Check sheet for the modelled part. Datum: model origin and axes. Units: mm. Face numbers are marked on the shaded views. A direction names the side the tool comes from. Round coordinates to 2 decimals unless told otherwise and drop trailing zeros. Order: outer loops, then holes, each group sorted by start corner. A loop starts at its lowest first (then second) coordinate and runs counter-clockwise, first axis right, second up.
(1) Tool access check on the marked faces 5, 6 and 7. Record the directions out of +Z, -Z, +X, -X, +Y, -Y that give a thin tool (end or side, any length) a straight path to the whole face; none if there is none.
(2) Depth check by flat-ended pin: pin 1 (1.6 mm diameter, centred on y = 25.5, z = 2, fed in from +X); pin 2 (10 mm diameter, centred on x = 16, y = 19.5, fed in from -Z); pin 3 (3 mm diameter, centred on x = 19, y = 28, fed in from +Z); pin 4 (1.6 mm diameter, centred on x = 7, y = -6, fed in from -Z). Enter the tip coordinate at first touch or a pass-through.
(3) Mould release check, pull along Y, two halves, no side actions. Record for the marked faces 1, 2, 3 and 4: released by +Y, released by -Y, zero draft, split by the parting line, or undercut.
(4) Sectioned sample at D-D, the plane z = 7.25. Enter the section's corners in (x, y), and give its area (3 significant figures).
(5) Sectioned sample at C-C, the plane x = 12.5. Enter the section's corners in (y, z).
(6) Thickness scan on probe 1 along Y at (x, z) = (13, 4.1); probe 2 along Y at (x, z) = (19.5, 3.4); probe 3 along Y at (x, z) = (17, 11). Record the ranges inside material, lowest first.
(7) Sectioned sample at B-B, the plane y = -5.5. Enter the section's corners in (x, z), and give its area (3 significant figures).
(8) Sectioned sample at A-A, the plane x = 6.5. Count the separate pieces of the cut face and the enclosed holes in it, and give its area (3 significant figures).
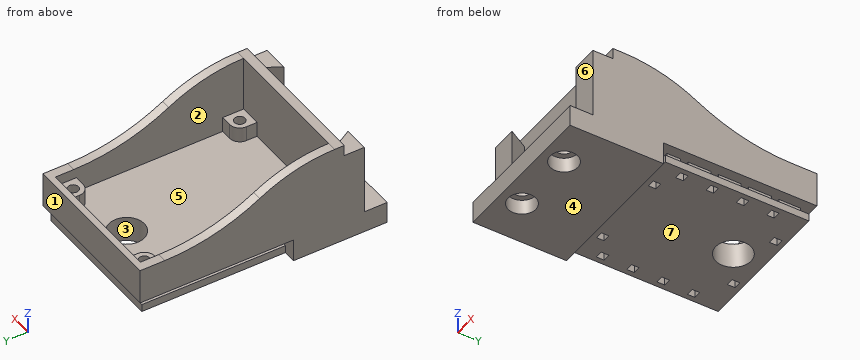
```python
from build123d import *

# Parameters (mm, degrees)
SKETCH2_W             = 30
SKETCH2_H             = 18.5
BOSS_EXTRUDE1_DEPTH   = 4.5
BOSS_EXTRUDE2_DEPTH   = 2
SKETCH4_W             = 26.3
SKETCH4_H             = 37.3
BOSS_EXTRUDE3_DEPTH   = 12
SKETCH5_W             = 30
SKETCH5_H             = 40.415903306
SKETCH5_W_2           = 26.3
SKETCH5_H_2           = 37.3
BOSS_EXTRUDE4_DEPTH   = 2
CUT_EXTRUDE1_DEPTH    = 53.877515324
SKETCH7_R             = 2.75
CUT_EXTRUDE2_DEPTH    = 3
SKETCH8_R             = 1.65
CUT_EXTRUDE3_DEPTH    = 51.656012741
SKETCH9_W             = 0.2
SKETCH9_H             = 4
TOLERANCE_CUT1_DEPTH  = 53.877515324
TOLERANCE_CUT2_DEPTH  = 0.2
BOSS_EXTRUDE5_DEPTH   = 3
SKETCH12_W            = 26.022193388
SKETCH12_H            = 26.438096694
BOSS_EXTRUDE6_DEPTH   = 1.5
SKETCH13_W            = 28.011096694
SKETCH13_H            = 28.427
BOSS_EXTRUDE7_DEPTH   = 1.5
SKETCH14_R            = 3.5
CUT_EXTRUDE6_DEPTH    = 50.555843518
SKETCH15_R            = 1.05
PCB_MOUNT_HOLES_DEPTH = 5
SKETCH16_W            = 1.5
SKETCH16_H            = 1.5
CUT_EXTRUDE8_DEPTH    = 3


with BuildPart() as part:
    # Sketch2 → Boss-Extrude1 (new body)
    with BuildSketch(Plane.XY):
        with Locations((13, -1.25)):
            Rectangle(SKETCH2_W, SKETCH2_H)
    extrude(amount=BOSS_EXTRUDE1_DEPTH)

    # Sketch3 → Boss-Extrude2 (add)
    with BuildSketch(Plane.XY.offset(4.5)):
        Polygon((-2, 38.415903306), (28, 38.415903306), (28, -6), (22.890598923, -6), (25.2, -2), (0.7, -2), (3.009401077, -6), (-2, -6), align=None)
    extrude(amount=BOSS_EXTRUDE2_DEPTH)

    # Sketch4 → Boss-Extrude3 (add)
    with BuildSketch(Plane.XY.offset(6.5)):
        Polygon((-2, 38.415903306), (-2, -6), (3.009401077, -6), (0.7, -2), (25.2, -2), (22.890598923, -6), (28, -6), (28, 38.415903306), align=None)
        with Locations((13, 18.5)):
            Rectangle(SKETCH4_W, SKETCH4_H, mode=Mode.SUBTRACT)
    extrude(amount=BOSS_EXTRUDE3_DEPTH)

    # Sketch5 → Boss-Extrude4 (add)
    with BuildSketch(Plane.XY.offset(18.5)):
        with Locations((13, 18.207951653)):
            Rectangle(SKETCH5_W, SKETCH5_H)
        with Locations((13, 18.5)):
            Rectangle(SKETCH5_W_2, SKETCH5_H_2, mode=Mode.SUBTRACT)
    extrude(amount=BOSS_EXTRUDE4_DEPTH)

    # Sketch6 → Cut-Extrude1 (cut, through all)
    with BuildSketch(Plane(origin=(28, 0, 0), x_dir=(0, 0, -1), z_dir=(1, 0, 0))):
        with BuildLine():
            Line((-11.5, 38.415903306), (-29.920257518, 38.415903306))
            Line((-29.920257518, 38.415903306), (-29.920257518, -0.15))
            Line((-29.920257518, -0.15), (-20.5, -0.15))
            ThreePointArc((-20.5, -0.15), (-19.490822016, 7.533583379), (-16.531743455, 14.695967606))
            ThreePointArc((-16.531743455, 14.695967606), (-12.779636198, 23.777860258), (-11.5, 33.520632668))
            Line((-11.5, 33.520632668), (-11.5, 38.415903306))
        make_face()
    extrude(amount=-CUT_EXTRUDE1_DEPTH, mode=Mode.SUBTRACT)

    # Sketch7 → Cut-Extrude2 (cut)
    with BuildSketch(Plane(origin=(0, 0, 0), x_dir=(-1, 0, 0), z_dir=(0, 0, -1))):
        with Locations((-19.5, -6.25)):
            Circle(SKETCH7_R)
        with Locations(Location((-6.5, -6.25, 0), (0, 0, 180))):
            Circle(SKETCH7_R)
    extrude(amount=-CUT_EXTRUDE2_DEPTH, mode=Mode.SUBTRACT)

    # Sketch8 → Cut-Extrude3 (cut, through all)
    with BuildSketch(Plane(origin=(0, 0, 3), x_dir=(-1, 0, 0), z_dir=(0, 0, -1))):
        with Locations((-19.5, -6.25)):
            Circle(SKETCH8_R)
        with Locations((-6.5, -6.25)):
            Circle(SKETCH8_R)
    extrude(amount=-CUT_EXTRUDE3_DEPTH, mode=Mode.SUBTRACT)

    # Sketch9 → tolerance_cut1 (cut, through all)
    with BuildSketch(Plane.ZY.offset(2)):
        with Locations((18.4, -4)):
            Rectangle(SKETCH9_W, SKETCH9_H)
    extrude(amount=-TOLERANCE_CUT1_DEPTH, mode=Mode.SUBTRACT)

    # Sketch10 → tolerance_cut2 (cut)
    with BuildSketch(Plane.XY.offset(4.5)):
        Polygon((28, -6), (22.890598923, -6), (25.2, -2), (0.7, -2), (3.009401077, -6), (-2, -6), (-2, -10.5), (28, -10.5), align=None)
    extrude(amount=-TOLERANCE_CUT2_DEPTH, mode=Mode.SUBTRACT)

    # Sketch11 → Boss-Extrude5 (add)
    with BuildSketch(Plane.XY.offset(6.5)):
        with BuildLine():
            Line((4, 35), (4, 37.15))
            Line((4, 37.15), (-0.15, 37.15))
            Line((-0.15, 37.15), (-0.15, 33))
            Line((-0.15, 33), (2, 33))
            ThreePointArc((2, 33), (3.414213562, 33.585786438), (4, 35))
        make_face()
        with BuildLine():
            Line((26.15, 33), (24, 33))
            ThreePointArc((24, 33), (22.585786438, 33.585786438), (22, 35))
            Line((22, 35), (22, 37.15))
            Line((22, 37.15), (26.15, 37.15))
            Line((26.15, 37.15), (26.15, 33))
        make_face()
        with BuildLine():
            Line((26.15, 4), (24, 4))
            ThreePointArc((24, 4), (22.585786438, 3.414213562), (22, 2))
            Line((22, 2), (22, -0.15))
            Line((22, -0.15), (26.15, -0.15))
            Line((26.15, -0.15), (26.15, 4))
        make_face()
        with BuildLine():
            Line((-0.15, 4), (2, 4))
            ThreePointArc((2, 4), (3.414213562, 3.414213562), (4, 2))
            Line((4, 2), (4, -0.15))
            Line((4, -0.15), (-0.15, -0.15))
            Line((-0.15, -0.15), (-0.15, 4))
        make_face()
    extrude(amount=BOSS_EXTRUDE5_DEPTH)

    # Sketch12 → Boss-Extrude6 (add)
    with BuildSketch(Plane(origin=(0, 0, 4.5), x_dir=(-1, 0, 0), z_dir=(0, 0, -1))):
        with Locations((-13, 23.207951653)):
            Rectangle(SKETCH12_W, SKETCH12_H)
    extrude(amount=BOSS_EXTRUDE6_DEPTH)

    # Sketch13 → Boss-Extrude7 (add)
    with BuildSketch(Plane(origin=(0, 0, 3), x_dir=(-1, 0, 0), z_dir=(0, 0, -1))):
        with Locations((-13, 23.207951653)):
            Rectangle(SKETCH13_W, SKETCH13_H)
    extrude(amount=BOSS_EXTRUDE7_DEPTH)

    # Sketch14 → Cut-Extrude6 (cut, through all)
    with BuildSketch(Plane.XY.offset(6.5)):
        with Locations((13, 31.463)):
            Circle(SKETCH14_R)
    extrude(amount=-CUT_EXTRUDE6_DEPTH, mode=Mode.SUBTRACT)

    # Sketch15 → pcb_mount_holes (cut)
    with BuildSketch(Plane.XY.offset(9.5)):
        with Locations((2, 35)):
            Circle(SKETCH15_R)
        with Locations((24, 35)):
            Circle(SKETCH15_R)
        with Locations((24, 2)):
            Circle(SKETCH15_R)
        with Locations((2, 2)):
            Circle(SKETCH15_R)
    extrude(amount=-PCB_MOUNT_HOLES_DEPTH, mode=Mode.SUBTRACT)

    # Sketch16 → Cut-Extrude8 (cut)
    with BuildSketch(Plane(origin=(0, 0, 1.5), x_dir=(-1, 0, 0), z_dir=(0, 0, -1))):
        with Locations((-25.261096694, 25.419380652)):
            Rectangle(SKETCH16_W, SKETCH16_H)
        with Locations((-25.261096694, 31.419380652)):
            Rectangle(SKETCH16_W, SKETCH16_H)
        with Locations((-25.261096694, 19.419380652)):
            Rectangle(SKETCH16_W, SKETCH16_H)
        with Locations((-25.261096694, 13.419380652)):
            Rectangle(SKETCH16_W, SKETCH16_H)
        with Locations((-21.014935628, 10.738903306)):
            Rectangle(SKETCH16_W, SKETCH16_H)
        with Locations((-19.514935628, 35.677)):
            Rectangle(SKETCH16_W, SKETCH16_H)
        with Locations((-4.985064372, 10.738903306)):
            Rectangle(SKETCH16_W, SKETCH16_H)
        with Locations((-0.738903306, 13.419380652)):
            Rectangle(SKETCH16_W, SKETCH16_H)
        with Locations((-0.738903306, 19.419380652)):
            Rectangle(SKETCH16_W, SKETCH16_H)
        with Locations((-0.738903306, 25.419380652)):
            Rectangle(SKETCH16_W, SKETCH16_H)
        with Locations((-0.738903306, 31.419380652)):
            Rectangle(SKETCH16_W, SKETCH16_H)
        with Locations((-6.485064372, 35.677)):
            Rectangle(SKETCH16_W, SKETCH16_H)
    extrude(amount=-CUT_EXTRUDE8_DEPTH, mode=Mode.SUBTRACT)


solid = part.part
```
Derived:
1. face 5: +Z
1. face 6: +Z, +X, -X, -Y
1. face 7: -Z, +X, -X, +Y
2. pin 1: stops at x = 27.01
2. pin 2: stops at z = 1.5
2. pin 3: stops at z = 6.5
2. pin 4: passes through
3. face 1: released by +Y
3. face 2: undercut
3. face 3: undercut
3. face 4: zero draft
4. outline: (-2, -6) - (3.01, -6) - (0.7, -2) - (25.2, -2) - (22.89, -6) - (28, -6) - (28, 38.42) - (-2, 38.42) - close; hole (-0.15, 4) - (2, 4) arc R2 cw to (4, 2) - (4, -0.15) - (22, -0.15) - (22, 2) arc R2 cw to (24, 4) - (26.15, 4) - (26.15, 33) - (24, 33) arc R2 cw to (22, 35) - (22, 37.15) - (4, 37.15) - (4, 35) arc R2 cw to (2, 33) - (-0.15, 33) - close; hole circle Ø2.1 at (2, 2); hole circle Ø2.1 at (2, 35); hole circle Ø2.1 at (24, 2); hole circle Ø2.1 at (24, 35)
4. area: 314 mm2
5. outline: (-10.5, 0) - (8, 0) - (8, 4.5) - (9.99, 4.5) - (9.99, 3) - (8.99, 3) - (8.99, 1.5) - (28, 1.5) - (28, 6.5) - (-0.15, 6.5) - (-0.15, 20.5) - (-2, 20.5) - (-2, 4.3) - (-10.5, 4.3) - close; (34.93, 1.5) - (37.42, 1.5) - (37.42, 3) - (36.43, 3) - (36.43, 4.5) - (38.42, 4.5) - (38.42, 11.5) - (37.15, 11.5) - (37.15, 6.5) - (34.93, 6.5) - close
6. probe 1: y = -10.5 to 8, 9.99 to 27.96, 34.96 to 36.43
6. probe 2: y = -10.5 to -7.9, -4.6 to 8, 9.99 to 34.93
6. probe 3: y = -2 to -0.15, 37.15 to 38.42
7. outline: (-2, 0) - (3.85, 0) - (3.85, 3) - (5.03, 3) - (5.03, 4.3) - (2.72, 4.3) - (2.72, 18.3) - (-2, 18.3) - close; (7.97, 3) - (9.15, 3) - (9.15, 0) - (16.85, 0) - (16.85, 3) - (18.03, 3) - (18.03, 4.3) - (7.97, 4.3) - close; (20.97, 3) - (22.15, 3) - (22.15, 0) - (28, 0) - (28, 18.3) - (23.18, 18.3) - (23.18, 4.3) - (20.97, 4.3) - close
7. area: 223 mm2
8. separate pieces: 3
8. enclosed holes: 0
8. area: 252 mm2
